Can you work these out from the model? Positions are in its coordinate system, mm. A direction names the side the tool comes from. Give positions to 0.01 mm unless a question says otherwise; leave off trailing zeros. Order: outer loops, then holes, each group sorted by start corner. A loop starts at its lowest first (then second) coordinate and runs counter-clockwise, first axis right, second up. Notation, with made-up numbers: (26.25, 4.5) - (58.25, 4.5) arc R15 ccw to (58.25, 16.5) - close; hole circle Ø8 at (-6, 53.25). An arc over 180 degrees is marked (long way). Answer as CSV lines item,"result".
```python
from build123d import *

# Parameters (mm, degrees)
SKETCH1_W               = 8
SKETCH1_H               = 8
BOSS_EXTRUDE1_DEPTH     = 3
CUT_EXTRUDE1_DEPTH      = 12.704699911
CUT_EXTRUDE1_DEPTH_BACK = 12.704699911
CUT_EXTRUDE2_DEPTH      = 11
SKETCH4_R               = 1.75
CUT_EXTRUDE3_DEPTH      = 0.4
SKETCH5_W               = 8
SKETCH5_H               = 1
BOSS_EXTRUDE2_DEPTH     = 2
FILLET1_R               = 4
CUT_EXTRUDE4_DEPTH      = 0.4
CUT_EXTRUDE5_DEPTH      = 0.5


with BuildPart() as part:
    # Sketch1 → Boss-Extrude1 (new body)
    with BuildSketch(Plane(origin=(0, 0, 0), x_dir=(1, 0, 0), z_dir=(0, 1, 0))):
        with Locations((4, 4)):
            Rectangle(SKETCH1_W, SKETCH1_H)
    extrude(amount=BOSS_EXTRUDE1_DEPTH)

    # Sketch2 → Cut-Extrude1 (cut, two sides: drawn at the far end of the back side and taken through both)
    with BuildSketch(Plane.XY.offset(-CUT_EXTRUDE1_DEPTH_BACK)):
        Polygon((0, 0), (0.6, 3), (0, 3), align=None)
        Polygon((8, 0), (7.4, 3), (8, 3), align=None)
    extrude(amount=CUT_EXTRUDE1_DEPTH + CUT_EXTRUDE1_DEPTH_BACK, mode=Mode.SUBTRACT)

    # Sketch3 → Cut-Extrude2 (cut)
    with BuildSketch(Plane(origin=(0, 0, 0), x_dir=(0, 0, -1), z_dir=(1, 0, 0))):
        Polygon((0, 0), (0.6, 3), (0, 3), align=None)
        Polygon((8, 3), (7.4, 3), (8, 0), align=None)
    extrude(amount=CUT_EXTRUDE2_DEPTH, mode=Mode.SUBTRACT)

    # Sketch4 → Cut-Extrude3 (cut)
    with BuildSketch(Plane.XZ):
        with Locations(Location((4, -3.75, 0), (0, 0, 270))):
            Circle(SKETCH4_R)
    extrude(amount=-CUT_EXTRUDE3_DEPTH, mode=Mode.SUBTRACT)

    # Sketch5 → Boss-Extrude2 (add)
    with BuildSketch(Plane.XZ):
        with Locations((4, -7.5)):
            Rectangle(SKETCH5_W, SKETCH5_H)
    extrude(amount=BOSS_EXTRUDE2_DEPTH)

    # Fillet1
    # the kernel refuses this fillet: 4 mm, written as the material it takes off along each edge
    with BuildSketch(Plane(origin=(8, -2, -16.660254038), x_dir=(0, 1, 0), z_dir=(0, 0, 1)), Plane(origin=(0, -2, 1.660254038), x_dir=(0, 1, 0), z_dir=(0, 0, -1))) as fillet1_piece_1:
        with BuildLine():
            CenterArc((4, 3.464101615), FILLET1_R, 180, 60)
            Line((0, 3.464101615), (-0.08, 3.464101615))
            Line((-0.08, 3.464101615), (-0.08, 0))
            Line((-0.08, 0), (0, -0.08))
            ThreePointArc((0, -0.08), (1, -0.08), (1.96, -0.069282032))
            Line((1.96, -0.069282032), (2, 0))
        make_face()
    extrude(amount=18.320508076, mode=Mode.SUBTRACT)

    # Sketch6 → Cut-Extrude4 (cut)
    with BuildSketch(Plane(origin=(0, 3, 0), x_dir=(1, 0, 0), z_dir=(0, 1, 0))):
        Polygon((2.358967796, 2.025988971), (1.401435745, 6.025988971), (2.189897284, 6.025988971), (2.811692155, 3.278392817), (3.469544719, 6.025988971), (4.519224207, 6.025988971), (5.170666514, 3.231918458), (5.790858822, 6.025988971), (6.580922925, 6.025988971), (5.641019078, 2.025988971), (4.688294719, 2.025988971), (3.991179335, 5.016373586), (3.275634463, 2.025988971), align=None)
    extrude(amount=-CUT_EXTRUDE4_DEPTH, mode=Mode.SUBTRACT)

    # Sketch7 → Cut-Extrude5 (cut)
    with BuildSketch(Plane(origin=(0, 3, 0), x_dir=(1, 0, 0), z_dir=(0, 1, 0))):
        with BuildLine():
            Line((7.025079926, 1.261869909), (7.025079926, 0.954177602))
            Line((7.025079926, 0.954177602), (5.978926079, 0.954177602))
            add(Edge.make_bspline(
                [(5.978926079, 0.954177602), (5.982468114, 0.980474374), (5.989550197, 1.033053173), (6.011445466, 1.109857564), (6.040668149, 1.184805528), (6.072383822, 1.245794978), (6.103928572, 1.294889387), (6.132549124, 1.335117725), (6.166692393, 1.37791895), (6.205862922, 1.423638586), (6.249844239, 1.472419552), (6.298964472, 1.524080492), (6.353457933, 1.578374089), (6.391795053, 1.615242112), (6.411618387, 1.634305807)],
                knots=[0, 0, 0, 0, 1.156289446, 2.311930546, 3.473459201, 4.661751613, 5.303057008, 6.018253237, 6.81459331, 7.690699809, 8.644447906, 9.679642995, 10.800191253, 12, 12, 12, 12], degree=3))
            add(Edge.make_bspline(
                [(6.411618387, 1.634305807), (6.427437635, 1.649575712), (6.457552822, 1.678645113), (6.500436909, 1.720271317), (6.538136439, 1.758537631), (6.571439659, 1.79245241), (6.599577217, 1.822879209), (6.622919237, 1.849340182), (6.641761343, 1.871943086), (6.651966244, 1.886282382), (6.656490182, 1.89263914)],
                knots=[0, 0, 0, 0, 1.480720495, 2.818855715, 4.024636094, 5.098235712, 6.019786162, 6.815086302, 7.474715479, 8, 8, 8, 8], degree=3))
            add(Edge.make_bspline(
                [(6.656490182, 1.89263914), (6.665754103, 1.908027503), (6.683623134, 1.937709873), (6.703218009, 1.984385935), (6.714979583, 2.031052356), (6.71659359, 2.062234592), (6.717387618, 2.077575038)],
                knots=[0, 0, 0, 0, 1.0911822, 2.104764037, 3.067617678, 4, 4, 4, 4], degree=3))
            add(Edge.make_bspline(
                [(6.717387618, 2.077575038), (6.716811351, 2.093538834), (6.7157211, 2.123741092), (6.706579153, 2.166362064), (6.690367393, 2.203000826), (6.668046783, 2.233769843), (6.639822327, 2.257877251), (6.606827118, 2.275690284), (6.568578157, 2.285538571), (6.541694532, 2.286833928), (6.527644028, 2.287510935)],
                knots=[0, 0, 0, 0, 1.193122327, 2.257294386, 3.237245624, 4.168877528, 5.075331632, 5.990371598, 6.949684428, 8, 8, 8, 8], degree=3))
            add(Edge.make_bspline(
                [(6.527644028, 2.287510935), (6.513688449, 2.286878661), (6.486729282, 2.285657243), (6.448414457, 2.274987105), (6.414896057, 2.256515974), (6.391009062, 2.235466338), (6.374872264, 2.214997095), (6.363877213, 2.197159499), (6.354400337, 2.17689052), (6.346003035, 2.154418352), (6.339370115, 2.129485554), (6.334028373, 2.102282013), (6.329723702, 2.072661336), (6.328354741, 2.052055079), (6.327644028, 2.041357089)],
                knots=[0, 0, 0, 0, 1.402788338, 2.709884207, 3.961032948, 5.225417836, 5.883680772, 6.578928686, 7.329201998, 8.132101139, 8.990263233, 9.922304639, 10.921339128, 12, 12, 12, 12], degree=3))
            Line((6.327644028, 2.041357089), (6.01995172, 2.071485294))
            add(Edge.make_bspline(
                [(6.01995172, 2.071485294), (6.022425519, 2.092258403), (6.027221819, 2.132534142), (6.039191066, 2.190383991), (6.054349674, 2.243753088), (6.073420305, 2.292542389), (6.095614746, 2.337062147), (6.122065099, 2.376644317), (6.15184716, 2.411727355), (6.184986668, 2.44229259), (6.221272944, 2.468437258), (6.259348879, 2.491775386), (6.299958585, 2.510920071), (6.342654946, 2.526698167), (6.387418668, 2.539307895), (6.434456788, 2.547645276), (6.483479006, 2.553509822), (6.516941776, 2.553951654), (6.534054285, 2.554177602)],
                knots=[0, 0, 0, 0, 1.270971563, 2.464210789, 3.586263665, 4.638946707, 5.643716971, 6.603612468, 7.52484387, 8.434700188, 9.336036235, 10.239171475, 11.145359471, 12.059630629, 13.003312604, 13.96741569, 14.960557767, 16, 16, 16, 16], degree=3))
            add(Edge.make_bspline(
                [(6.534054285, 2.554177602), (6.552657792, 2.553820052), (6.58889046, 2.553123679), (6.641783721, 2.547373025), (6.69147314, 2.537345926), (6.738393137, 2.524063615), (6.782061867, 2.506330758), (6.82284322, 2.484892472), (6.860095371, 2.458935129), (6.894373612, 2.429874295), (6.925015616, 2.397916799), (6.95185524, 2.363828728), (6.974341388, 2.327633829), (6.993210719, 2.289773279), (7.007221071, 2.249637846), (7.017429622, 2.207782494), (7.024198302, 2.164011958), (7.024782801, 2.134117674), (7.025079926, 2.118921192)],
                knots=[0, 0, 0, 0, 1.210756838, 2.35810096, 3.457354827, 4.507168606, 5.527358126, 6.519769748, 7.499700793, 8.476517721, 9.440526811, 10.376769937, 11.295256217, 12.209626307, 13.124630862, 14.055668209, 15.011616881, 16, 16, 16, 16], degree=3))
            add(Edge.make_bspline(
                [(7.025079926, 2.118921192), (7.024688468, 2.101480457), (7.023911876, 2.066880717), (7.016476584, 2.015731964), (7.005116907, 1.965762694), (6.988328197, 1.916850789), (6.967047205, 1.867822963), (6.939615495, 1.818569171), (6.907765206, 1.767604004), (6.882827684, 1.7346528), (6.86995172, 1.71763914)],
                knots=[0, 0, 0, 0, 0.953409949, 1.89141903, 2.821310783, 3.752688675, 4.715703262, 5.740811754, 6.833515735, 8, 8, 8, 8], degree=3))
            add(Edge.make_bspline(
                [(6.86995172, 1.71763914), (6.865085171, 1.711509707), (6.854662151, 1.698381883), (6.836929855, 1.678252394), (6.816379649, 1.656264646), (6.793301796, 1.632007081), (6.766933989, 1.606338723), (6.738224942, 1.578186143), (6.705911376, 1.548989439), (6.672442351, 1.518020294), (6.638827847, 1.487878461), (6.607931272, 1.459250402), (6.579866901, 1.433920718), (6.555941744, 1.410491095), (6.534748531, 1.390560588), (6.517051134, 1.373107183), (6.502518393, 1.358553413), (6.482493212, 1.335867777), (6.457013442, 1.305185447), (6.439087381, 1.275867612), (6.430528644, 1.261869909)],
                knots=[0, 0, 0, 0, 0.665555651, 1.425465941, 2.280616993, 3.225313414, 4.272635571, 5.410053715, 6.644756443, 7.976022804, 9.288331007, 10.484517221, 11.558462543, 12.503158964, 13.33222979, 14.032602617, 14.617328242, 15.080653724, 16.606167857, 18, 18, 18, 18], degree=3))
            Line((6.430528644, 1.261869909), (7.025079926, 1.261869909))
        make_face()
    extrude(amount=-CUT_EXTRUDE5_DEPTH, mode=Mode.SUBTRACT)


solid = part.part
```
1) Which directions (+Z, -Z, +X, -X, +Y, -Y) give clear straight access to the entire face, cutting with the end or side of a thin tool? Please do faces 1 (the flat face through (1.887, 2.803, -3.998)), 2 (the flat face through (3, 0, -2)), 3 (the cylindrical face through (2.94, 0.2, -2.36)).
Answer block:
face 1,"+Y"
face 2,"+Z, +X, -X, -Y"
face 3,"-Y"
2) If we mould it in two halves opening along Z, with no side actions, what happens to faces 4 (the flat face through (3.9, 1.5, -0.3)), 5 (the flat face through (3.9, 1.5, -7.7)), 6 (the flat face through (0.3, 1.5, -4.1)), 7 (the flat face through (4, 0.4, -4))? For each: +Z half, -Z half, draft (parallel to the pull), parting line (faces both ways), or undercut.
Answer block:
face 4,"+Z half"
face 5,"-Z half"
face 6,"draft"
face 7,"undercut"
3) I need wall thicknesses on line 1 along Y through (x, z) = (1, -5); line 2 along Y through (x, z) = (2.25, -4.5); line 3 along X through (y, z) = (0.1, -3.75). Which ranges of each line are inside material? Lowest first, please. Write a range as [from, to].
Answer block:
line 1,"[0, 3]"
line 2,"[0, 2.6]"
line 3,"[0.02, 2.25], [5.75, 7.98]"
4) I want a section at C-C on y = 1.45. Write out the boundary of the cut face in (x, z).
Answer block:
outline,"(0.29, -7.71) - (7.71, -7.71) - (7.71, -0.29) - (0.29, -0.29) - close"
5) I want a section at A-A on x = 3. Write out the boundary of the cut face in (y, z).
Answer block:
outline,"(-1.97, -8) - (0, -8) - (3, -7.4) - (3, -4.06) - (2.6, -4.06) - (2.6, -2.03) - (3, -2.03) - (3, -0.6) - (0, 0) - (0, -2.31) - (0.4, -2.31) - (0.4, -5.19) - (0, -5.19) - (0, -7) - (-1.97, -7) - close"
6) I want a section at B-B on z = -2.75. Write out the boundary of the cut face in (x, y), plus the area to 3 significant figures.
Answer block:
outline,"(0, 0) - (2.56, 0) - (2.56, 0.4) - (5.44, 0.4) - (5.44, 0) - (8, 0) - (7.4, 3) - (5.81, 3) - (5.81, 2.6) - (4.52, 2.6) - (4.52, 3) - (3.45, 3) - (3.45, 2.6) - (2.19, 2.6) - (2.19, 3) - (0.6, 3) - close"
area,"20.0 mm2"
7) I want a section at D-D on z = -3.75. Write out the boundary of the cut face in (x, y), plus the area to 3 significant figures.
Answer block:
outline,"(0, 0) - (2.25, 0) - (2.25, 0.4) - (5.75, 0.4) - (5.75, 0) - (8, 0) - (7.4, 3) - (6.05, 3) - (6.05, 2.6) - (5.29, 2.6) - (5.29, 3) - (5.05, 3) - (5.05, 2.6) - (4.29, 2.6) - (4.29, 3) - (3.69, 3) - (3.69, 2.6) - (2.92, 2.6) - (2.92, 3) - (2.7, 3) - (2.7, 2.6) - (1.95, 2.6) - (1.95, 3) - (0.6, 3) - close"
area,"19.6 mm2"
8) I'm going to push flat-ended pins straight in: P1, Ø0.6, axis at x = 5.5, y = -1, coming from the +Z side; P2, Ø2, axis at x = 4, z = -3.75, coming from the -Y side; P3, Ø4, axis at x = 3.5, z = -3.5, coming from the -Y side. Where does each tip first touch, or does it pass through?
Answer block:
P1,"z = -7"
P2,"y = 0.4"
P3,"y = 0"
